Input: part model. Units: mm. Frame: model coordinates. Face numbers are marked on the shaded views. A direction names the side the tool comes from. Give positions to 0.01 mm unless a question says otherwise; leave off trailing zeros. Write each loop counter-clockwise with the first axis right and the second up, starting at its lowest first coordinate (ties: lowest second). Pieces come first, ordered by that corner, then holes.
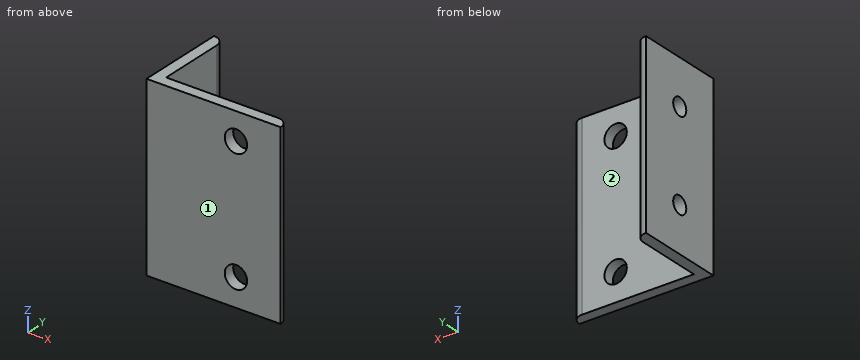
```python
from build123d import *

# Parameters (mm, degrees)
BOSS_EXTRUDE1_DEPTH              = 25.4
F_1_4_0_25_DIAMETER_HOLE1_D      = 6.35
F_1_4_0_25_DIAMETER_HOLE1_DEPTH  = 17.526
F_1_4_0_25_DIAMETER_HOLE1_TIP    = 1.907732465
F_10_0_1935_DIAMETER_HOLE1_D     = 4.9149
F_10_0_1935_DIAMETER_HOLE1_DEPTH = 17.526
F_10_0_1935_DIAMETER_HOLE1_TIP   = 1.476584928
FILLET1_R                        = 3.175


with BuildPart() as part:
    # Sketch1 → Boss-Extrude1 (new, symmetric)
    with BuildSketch(Plane.XY):
        Polygon((-8.126488095, 19.768154762), (-8.126488095, -5.631845238), (29.973511905, -5.631845238), (29.973511905, -2.456845238), (-4.951488095, -2.456845238), (-4.951488095, 19.768154762), align=None)
    extrude(amount=BOSS_EXTRUDE1_DEPTH, both=True)

    # 1/4 (0.25) Diameter Hole1
    with Locations(Plane(origin=(0, -2.456845238, 0), x_dir=(1, 0, 0), z_dir=(0, 1, 0))):
        with Locations((17.273511905, 17.4625), (17.273511905, -17.5895)):
            Hole(F_1_4_0_25_DIAMETER_HOLE1_D / 2, depth=F_1_4_0_25_DIAMETER_HOLE1_DEPTH)
            with Locations((0, 0, -(F_1_4_0_25_DIAMETER_HOLE1_DEPTH + F_1_4_0_25_DIAMETER_HOLE1_TIP / 2))):  # 118° drill point
                Cone(0, F_1_4_0_25_DIAMETER_HOLE1_D / 2, F_1_4_0_25_DIAMETER_HOLE1_TIP, mode=Mode.SUBTRACT)

    # #10 (0.1935) Diameter Hole1
    with Locations(Plane(origin=(-4.951488095, 0, 0), x_dir=(0, 0, -1), z_dir=(1, 0, 0))):
        with Locations((12.7, 7.068154762), (-12.7, 7.068154762)):
            Hole(F_10_0_1935_DIAMETER_HOLE1_D / 2, depth=F_10_0_1935_DIAMETER_HOLE1_DEPTH)
            with Locations((0, 0, -(F_10_0_1935_DIAMETER_HOLE1_DEPTH + F_10_0_1935_DIAMETER_HOLE1_TIP / 2))):  # 118° drill point
                Cone(0, F_10_0_1935_DIAMETER_HOLE1_D / 2, F_10_0_1935_DIAMETER_HOLE1_TIP, mode=Mode.SUBTRACT)

    # Fillet1
    fillet1_edges = [part.edges().sort_by_distance(p)[0] for p in [
        (29.973511905, -2.456845238, 0),
        (-4.951488095, 19.768154762, 0),
    ]]
    fillet(fillet1_edges, radius=FILLET1_R - 0.0001)  # a hair under: the kernel refuses the full size


solid = part.part
```
Q1. Section C-C, the plane y = 5.5. Return the cut outline in (x, z), then the cut area to 3 significant figures.
Q2. Material intervals for line 1 along X through (y, z) = (11, -16); line 2 along Y through (x, z) = (7, 7); line 3 along Y through (x, z) = (-7.35, 12.7), sorted ascending.
Q3. Pin query (flat end, axial travel): pin 1 (12 mm diameter, centred on x = 18, y = 9.5, fed in from +Z); pin 2 (15 mm diameter, centred on y = 9, z = 11, fed in from +X); pin 3 (10 mm diameter, centred on x = 17.27, z = 17.59, fed in from +Y). Return the tip coordinate at first contact, or that it passes through.
Q4. Access query for the marked faces 1 and 2. Directions: +Z, -Z, +X, -X, +Y, -Y. A direction counts if a zero-diameter tool reaches every point of the face in a straight line with its end or side. Return the directions, or none.
Q5. Section D-D, the plane x = 17.5. Return the cut outline in (y, z).
Solutions:
1. outline: (-8.13, -25.4) - (-4.95, -25.4) - (-4.95, -14.59) - (-8.13, -14.59) - close; (-8.13, -10.81) - (-4.95, -10.81) - (-4.95, 10.81) - (-8.13, 10.81) - close; (-8.13, 14.59) - (-4.95, 14.59) - (-4.95, 25.4) - (-8.13, 25.4) - close
1. area: 137 mm2
2. line 1: x = -8.13 to -4.95
2. line 2: y = -5.63 to -2.46
2. line 3: y = -5.63 to 4.61, 9.53 to 19.67
3. pin 1: passes through
3. pin 2: stops at x = -4.95
3. pin 3: stops at y = -2.46
4. face 1: +Z, -Z, +X, -X, -Y
4. face 2: +Z, -Z, +X, +Y
5. outline: (-5.63, -25.4) - (-2.46, -25.4) - (-2.46, -20.63) - (-5.63, -20.63) - close; (-5.63, -14.3) - (-2.46, -14.3) - (-2.46, 14.42) - (-5.63, 14.42) - close; (-5.63, 20.76) - (-2.46, 20.76) - (-2.46, 25.4) - (-5.63, 25.4) - close
